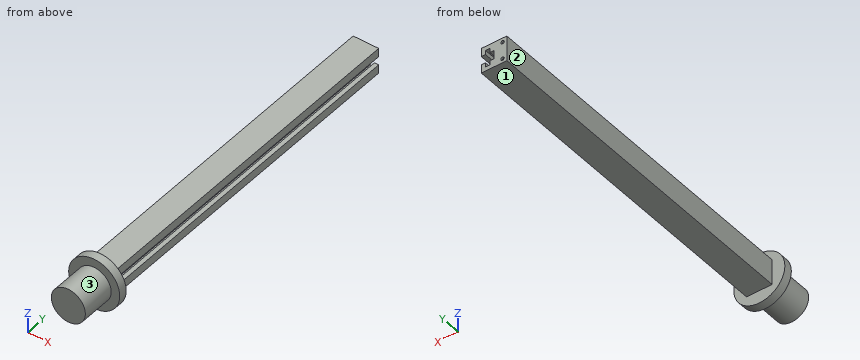
```python
from build123d import *

# Parameters (mm, degrees)
SKETCH5_W           = 150
SKETCH5_H           = 150
BOSS_EXTRUDE1_DEPTH = 2050
CUT_EXTRUDE1_DEPTH  = 2000
SKETCH8_R           = 10
CUT_EXTRUDE2_DEPTH  = 10


with BuildPart() as part:
    # Sketch4 → Revolve1 (revolve)
    with BuildSketch(Plane.XY, mode=Mode.PRIVATE) as revolve1_sk:
        Polygon((150, 101.851851852), (0, 101.851851852), (0, -148.148148148), (100, -148.148148148), (100, 51.851851852), (150, 51.851851852), align=None)
    revolve(revolve1_sk.sketch.rotate(Axis((0, 101.851851852, 0), (0, -1, 0)), 180), axis=Axis((0, 101.851851852, 0), (0, -1, 0)))

    # Sketch5 → Boss-Extrude1 (add)
    with BuildSketch(Plane(origin=(0, 101.851851852, 0), x_dir=(1, 0, 0), z_dir=(0, 1, 0))):
        Rectangle(SKETCH5_W, SKETCH5_H)
    extrude(amount=BOSS_EXTRUDE1_DEPTH)

    # Sketch6 → Cut-Extrude1 (cut)
    with BuildSketch(Plane(origin=(0, 2151.851851852, 0), x_dir=(1, 0, 0), z_dir=(0, 1, 0))):
        Polygon((0, 0), (0, 25), (25, 25), (25, 50), (50, 50), (50, 25), (75, 25), (75, -25), (50, -25), (50, -50), (25, -50), (25, -25), (0, -25), align=None)
    extrude(amount=-CUT_EXTRUDE1_DEPTH, mode=Mode.SUBTRACT)

    # Sketch8 → Cut-Extrude2 (cut)
    with BuildSketch(Plane(origin=(0, 2151.851851852, 0), x_dir=(1, 0, 0), z_dir=(0, 1, 0))):
        with Locations(Location((-50, 50, 0), (0, 0, 180))):
            Circle(SKETCH8_R)
        with Locations((-50, -50)):
            Circle(SKETCH8_R)
    extrude(amount=-CUT_EXTRUDE2_DEPTH, mode=Mode.SUBTRACT)


solid = part.part
```
Design review of the part built by this model. Coordinates are the model's own, in mm. Face numbers are marked on the shaded views. A direction names the side the tool comes from. Give positions to 0.01 mm unless a question says otherwise; leave off trailing zeros. Write each loop counter-clockwise with the first axis right and the second up, starting at its lowest first coordinate (ties: lowest second). Pieces come first, ordered by that corner, then holes. Notation, with made-up numbers: (-27.75, 7.25) -> (31.25, 7.25) arc R7 cw to (31.25, 20.25) -> close; hole circle Ø11 at (85, 29.5). An arc over 180 degrees is marked (long way). Answer in a Markdown table with one row per item.
(1) For the marked faces 1, 2 and 3, list the 3-axis set-ups (+Z, -Z, +X, -X, +Y, -Y) from which the entire face can be reached by the end or side of a thin tool; tool diameter is ignored.
Results:
| item | result |
|---|---|
| face 1 | -Z, +X, -X, +Y |
| face 2 | +Z, -Z, -X, +Y |
| face 3 | -Y |
(2) Consider section A-A (z = 0). State the section outline as (x, y) points.
Results:
| item | result |
|---|---|
| outline | (-150, 51.85) -> (-100, 51.85) -> (-100, -148.15) -> (100, -148.15) -> (100, 51.85) -> (150, 51.85) -> (150, 101.85) -> (75, 101.85) -> (75, 151.85) -> (0, 151.85) -> (0, 2151.85) -> (-75, 2151.85) -> (-75, 101.85) -> (-150, 101.85) -> close |
(3) To check wall thickness, follow probe 1 along Z at (x, y) = (-50, 2148); probe 2 along X at (y, z) = (939, -41); probe 3 along Z at (x, y) = (13.5, 880.5). State the ranges of each line that lie inside material, in increasing order.
Results:
| item | result |
|---|---|
| probe 1 | -75 to -60, -40 to 40, 60 to 75 |
| probe 2 | -75 to 25, 50 to 75 |
| probe 3 | -75 to -25, 25 to 75 |
(4) Clearance check with flat-ended pins moving along their axes: pin 1 (7.5 mm diameter, centred on x = 34.5, y = 1221.5, fed in from -Z); pin 2 (6 mm diameter, centred on y = 587.5, z = 37.5, fed in from -X); pin 3 (12.5 mm diameter, centred on y = 1044, z = -43.5, fed in from +X); pin 4 (10 mm diameter, centred on x = -46.5, z = 54, fed in from +Y). State where each tip first meets the part, or that it passes through.
Results:
| item | result |
|---|---|
| pin 1 | z = -75 |
| pin 2 | x = -75 |
| pin 3 | x = 75 |
| pin 4 | y = 2151.85 |
(5) Consider section B-B (y = 780.5). State the section outline as (x, z) points, then the cut area to 3 significant figures.
Results:
| item | result |
|---|---|
| outline | (-75, -75) -> (75, -75) -> (75, -25) -> (50, -25) -> (50, -50) -> (25, -50) -> (25, -25) -> (0, -25) -> (0, 25) -> (25, 25) -> (25, 50) -> (50, 50) -> (50, 25) -> (75, 25) -> (75, 75) -> (-75, 75) -> close |
| area | 17,500 mm2 |
(6) Consider section C-C (x = -19). State the section outline as (y, z) points, then the cut area to 3 significant figures.
Results:
| item | result |
|---|---|
| outline | (-148.15, -98.18) -> (51.85, -98.18) -> (51.85, -148.79) -> (101.85, -148.79) -> (101.85, -75) -> (2151.85, -75) -> (2151.85, 75) -> (101.85, 75) -> (101.85, 148.79) -> (51.85, 148.79) -> (51.85, 98.18) -> (-148.15, 98.18) -> close |
| area | 362,000 mm2 |
